Check sheet for the modelled part. Datum: model origin and axes. Units: mm. Give positions to 0.01 mm unless a question says otherwise; leave off trailing zeros. Loops run counter-clockwise (first coordinate to the right, second up) from the corner with the lowest first, then second, coordinate; pieces in that order, holes last.
Autodesk Inventor part; units mm, degrees
ref_plane "YZ Plane" through (0, 0, 0) normal (1, 0, 0) x (0, 1, 0)
ref_plane "XZ Plane" through (0, 0, 0) normal (0, 1, 0) x (-1, 0, 0)
ref_plane "XY Plane" through (0, 0, 0) normal (0, 0, 1) x (1, 0, 0)
ref_plane "Arbeitsebene1" through (0, 0, 0) normal (0, 0, 1) x (1, 0, 0)
sketch "Skizze1" plane through (0, 0, 0) normal (0, 0, 1) x (1, 0, 0)
  circle A0 centre (17.3893, 23.3893) radius 1.4
  circle A1 centre (-17.3893, -25.3893) radius 1.4
  circle A2 centre (17.3893, -25.3893) radius 1.4
  circle A3 centre (-17.3893, 23.3893) radius 1.4
  arc A4 (21, -31) -> (23, -29) centre (21, -29) ccw
  line L0 (23, -29) -> (23, 29)
  line L1 (11.5, 29) -> (23, 29)
  line L2 (11.5, 29) -> (11.5, -19)
  line L3 (11.5, -19) -> (-11.5, -19)
  line L4 (-11.5, -19) -> (-11.5, 29)
  line L5 (-23, 29) -> (-11.5, 29)
  line L6 (-23, 29) -> (-23, -29)
  arc A5 (-23, -29) -> (-21, -31) centre (-21, -29) ccw
  line L7 (-21, -31) -> (21, -31)
  circle A6 centre (-17.3893, -25.3893) radius 4
  circle A7 centre (17.3893, -25.3893) radius 4
  line L8 (-21, -31) -> (21, -31)
  line L9 (23, -29) -> (23, 2)
  line L10 (21, 4) -> (-21, 4)
  line L11 (-23, 2) -> (-23, -29)
  circle A8 centre (0, -6) radius 5.75
  arc A9 (-21, 4) -> (-23, 2) centre (-21, 2) ccw
  arc A10 (23, 2) -> (21, 4) centre (21, 2) ccw
  arc A11 (21, -31) -> (23, -29) centre (21, -29) ccw
  arc A12 (-23, -29) -> (-21, -31) centre (-21, -29) ccw
  point P0 (0, 0)
  point P1 (23, 4)
  dimension "d0" = 8
  dimension "d1" = 8
  dimension "d2" = 11.5
  dimension "d3" = 25
  dimension "d4" = 35
  dimension "d5" = 0
  dimension "d6" = 2
extrude "Extrusion1" add sketch "Skizze1" along normal blind 10 contours L7 A5 L6 A9 L10 L4 L3 L2 A10 L0 A4 | L2 L3 L4 L10
sketch "Skizze2" plane through (23, -29, 0) normal (1, 0, 0) x (0, 0, -1)
  line L0 (-10, 17.25) -> (0, 17.25)
  line L1 (-10, 28.75) -> (0, 28.75)
  line L2 (-10, 0) -> (-10, 31)
  line L3 (0, 0) -> (0, 31)
  circle A0 centre (-5, 23) radius 1.4
  point P0 (0, 29)
  dimension "d9" = 2.8
  dimension "d10" = 5.75
extrude "Extrusion2" cut sketch "Skizze2" against normal through all contours A0
sketch "Skizze3" plane through (-21, -31, 0) normal (0, -1, 0) x (1, 0, 0)
  line L0 (15.25, 10) -> (15.25, 0)
  line L1 (26.75, 10) -> (26.75, 0)
  circle A0 centre (21, 5) radius 1.4
  point P0 (21, 0)
  dimension "d13" = 2.8
extrude "Extrusion3" cut sketch "Skizze3" against normal through all
properties part number "Anglerfish_coverslipclamp_lampclamp"
(1) Release check for a two-part mould opening along X. For faces 1 (the face through (-22.4, -30.43, 4.93)), 2 (the face through (5.312, -3.798, 4.93)), 3 (the face through (-1.03, 1.76, 5.95)), 4 (the face through (14.41, -5.579, 3.665)) record: pulls with the +X half, pulls with the -X half, needs draft (parallel to the pull), parting line crosses it, or undercut.
(2) Material ranges on line 1 (X direction, y = -24, z = 7.25); line 2 (Z direction, x = -16.25, y = -6); line 3 (X direction, y = -23.5, z = 5) (3 decimals), recorded low to high.
(3) Section check D-D on x = 0. Record the boundary of the cut face in (y, z), plus the area to 3 significant figures.
(4) Section check C-C on z = 5. Record the boundary of the cut face in (x, y), plus the area to 3 significant figures.
(5) Section check B-B on x = -14. Record the boundary of the cut face in (y, z) (3 decimals).
(6) Section check A-A on y = -23. Record the boundary of the cut face in (x, z).
Computed values:
1. face 1: pulls with the -X half
1. face 2: undercut
1. face 3: undercut
1. face 4: needs draft
2. line 1: x = -23 to -21.14, -13.64 to 13.64, 21.14 to 23
2. line 2: z = 0 to 3.6, 6.4 to 10
2. line 3: x = -23 to -20.915, -13.864 to -1.4, 1.4 to 13.864, 20.915 to 23
3. outline: (-31, 0) - (-11.75, 0) - (-11.75, 3.6) - (-31, 3.6) - close; (-31, 6.4) - (-11.75, 6.4) - (-11.75, 10) - (-31, 10) - close; (-0.25, 0) - (4, 0) - (4, 3.6) - (-0.25, 3.6) - close; (-0.25, 6.4) - (4, 6.4) - (4, 10) - (-0.25, 10) - close
3. area: 169 mm2
4. outline: (-23, -29) arc R2 ccw to (-21, -31) - (-1.4, -31) - (-1.4, -11.58) arc R5.75 cw to (-5.58, -7.4) - (-23, -7.4) - close; (-23, -4.6) - (-5.58, -4.6) arc R5.75 cw to (-1.4, -0.42) - (-1.4, 4) - (-21, 4) arc R2 ccw to (-23, 2) - close; (1.4, -31) - (21, -31) arc R2 ccw to (23, -29) - (23, -7.4) - (5.58, -7.4) arc R5.75 cw to (1.4, -11.58) - close; (1.4, -0.42) arc R5.75 cw to (5.58, -4.6) - (23, -4.6) - (23, 2) arc R2 ccw to (21, 4) - (1.4, 4) - close; hole circle Ø8 at (-17.39, -25.39); hole circle Ø8 at (17.39, -25.39)
4. area: 1,240 mm2
5. outline: (-31, 0) - (-27.514, 0) - (-27.514, 10) - (-31, 10) - close; (-23.265, 0) - (4, 0) - (4, 10) - (-23.265, 10) - close; hole circle Ø2.8 at (-6, 5)
6. outline: (-23, 0) - (-20.6, 0) - (-20.6, 10) - (-23, 10) - close; (-14.18, 0) - (14.18, 0) - (14.18, 10) - (-14.18, 10) - close; (20.6, 0) - (23, 0) - (23, 10) - (20.6, 10) - close; hole circle Ø2.8 at (0, 5)
